Source: CAD feature listing. Evaluate the final solid. Frame: model axes, mm. Coordinates: 2 decimals unless noted, no trailing zeros. Loops run counter-clockwise (first coordinate to the right, second up) from the corner with the lowest first, then second, coordinate; pieces in that order, holes last.
Item 1: Line query: probe 1 along Z at (x, y) = (0, -12.75); probe 2 along Z at (x, y) = (-3.5, -17.75); probe 3 along X at (y, z) = (-6.75, -41.5). Output: solid intervals per line, ascending.
Item 2: Section query A-A, the plane x = 0. Return the cut outline in (y, z).
Item 3: Section query B-B, the plane z = 6. Return the cut outline in (x, y) (3 decimals).
Item 4: Pin query (flat end, axial travel): pin 1 Ø10 at (x, y) = (-9.5, -15) entering from +Z; pin 2 Ø1 at (y, z) = (-3, 43) entering from -X; pin 3 Ø1 at (y, z) = (-4.5, 1) entering from -X; pin 4 Ø8.5 at (x, z) = (0, -40.96) entering from -Y. Return the tip coordinate at first contact, or that it passes through.
Item 5: Section query C-C, the plane x = 20.5. Return the cut outline in (y, z).
```python
from build123d import *

# Parameters (mm, degrees)
F0_R     = 7.1501
F1_DEPTH = 25.4


with BuildPart() as f1:
    # F0 (on Front) → F1 (new body)
    with BuildSketch(Plane.XZ):
        with BuildLine():
            ThreePointArc((25.2923109526, 128.4121790948), (0.3078063491, 105.3504959458), (-25.2282585963, 127.7999076763))
            Line((-25.2282585963, 127.7999076763), (-15.8507982355, -41.8316227352))
            ThreePointArc((-15.8507982355, -41.8316227352), (-0.4382938581, -25.0864207714), (15.875, -40.9553691768))
            ThreePointArc((15.875, -40.9553691768), (15.8689095808, -41.3950664769), (15.8506429964, -41.8344263987))
            Line((15.8506429964, -41.8344263987), (25.2923109526, 128.4121790948))
        make_face()
        with BuildLine():
            ThreePointArc((25.3955649857, 130.273995114), (25.3988912222, 130.5113026086), (25.4, 130.7486308232))
            ThreePointArc((25.4, 130.7486308232), (0.0749748393, 156.1485201689), (-25.3995573837, 130.8985798486))
            Line((-25.3995573837, 130.8985798486), (-25.2282585963, 127.7999076763))
            ThreePointArc((-25.2282585963, 127.7999076763), (0.3078063491, 105.3504959458), (25.2923109526, 128.4121790948))
            Line((25.2923109526, 128.4121790948), (25.3955649857, 130.273995114))
        make_face()
        with Locations((0, 130.7486308232)):
            Circle(F0_R, mode=Mode.SUBTRACT)
        with BuildLine():
            ThreePointArc((15.875, -40.9553691768), (-0.4382938581, -25.0864207714), (-15.8507982355, -41.8316227352))
            ThreePointArc((-15.8507982355, -41.8316227352), (-0.001403979, -56.8303691147), (15.8506429964, -41.8344263987))
            ThreePointArc((15.8506429964, -41.8344263987), (15.8689095808, -41.3950664769), (15.875, -40.9553691768))
        make_face()
        with Locations((0, -40.9553691768)):
            Circle(F0_R, mode=Mode.SUBTRACT)
    extrude(amount=F1_DEPTH)


solid = f1.part
```
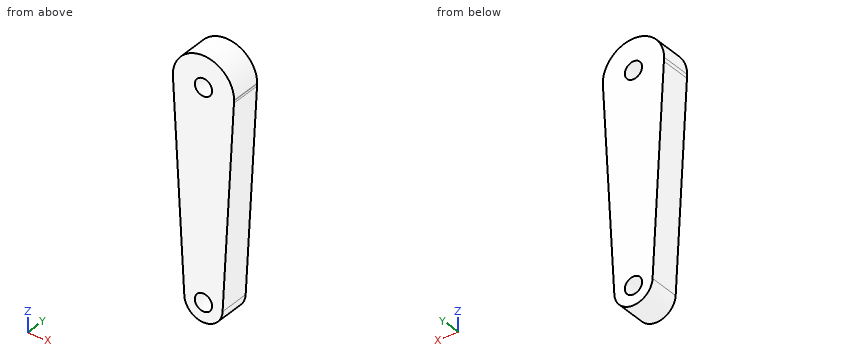
Verdict:
1. probe 1: z = -56.83 to -48.11, -33.81 to 123.6, 137.9 to 156.15
1. probe 2: z = -56.44 to -47.19, -34.72 to 124.51, 136.98 to 155.91
1. probe 3: x = -15.87 to -7.13, 7.13 to 15.87
2. outline: (-25.4, -56.83) - (0, -56.83) - (0, -48.11) - (-25.4, -48.11) - close; (-25.4, -33.81) - (0, -33.81) - (0, 123.6) - (-25.4, 123.6) - close; (-25.4, 137.9) - (0, 137.9) - (0, 156.15) - (-25.4, 156.15) - close
3. outline: (-18.495, -25.4) - (18.503, -25.4) - (18.503, 0) - (-18.495, 0) - close
4. pin 1: stops at z = 155.75
4. pin 2: stops at x = -20.57
4. pin 3: stops at x = -18.25
4. pin 4: passes through
5. outline: (-25.4, 42) - (0, 42) - (0, 145.75) - (-25.4, 145.75) - close
